Here's how the part is built. I have some questions about the finished solid (model axes, mm). Face numbers are marked on the shaded views. A direction names the side the tool comes from. Round coordinates to 2 decimals unless told otherwise and drop trailing zeros. Write each loop counter-clockwise with the first axis right and the second up, starting at its lowest first coordinate (ties: lowest second). Pieces come first, ordered by that corner, then holes. Notation, with made-up numbers: (62, 77.25) - (69, 77.25) arc R10 ccw to (69, 86.25) - close; hole circle Ø2 at (-28, 16.5). An arc over 180 degrees is marked (long way). One line per question, with ' | ' between items. Start each with the question number.
(1) Imagine slicing it at C-C (y = -6.5). Write out the boundary of the cut face in (x, z).
(2) Imagine slicing it at A-A (z = 1.7). Write out the boundary of the cut face in (x, y), plus the area to 3 significant figures.
(3) Imagine slicing it at D-D (y = -18). Write out the boundary of the cut face in (x, z), plus the area to 3 significant figures.
(4) For the marked faces 1, 2, 3 and 4, which set-ups out of +Z, -Z, +X, -X, +Y, -Y let a thin tool reach every point of the face, with its end or its side?
(5) Imagine slicing it at B-B (y = -12.5). Write out the boundary of the cut face in (x, z).
(6) If I drill on L1, parallel to Z at x = 0, y = -17.25; L2, parallel to Y at x = -1.25, z = 0.9; L3, parallel to Z at x = 3.25, y = 2, over which ranges is the centre line in solid material (lowest first)?
(7) Will these pins go through, and if not, where does the flat tip stop? pin 1 (2.5 mm diameter, centred on x = 0, y = 0, fed in from +Z); pin 2 (1 mm diameter, centred on x = -2, y = -6.5, fed in from +Z); pin 3 (1.8 mm diameter, centred on x = -1, z = -1.5, fed in from +Y); pin 4 (2 mm diameter, centred on y = -7.5, z = -1, fed in from -X).
(8) Thinking about a two-plate mould opening in Y: for the marked faces 5, 6, 7 and 8, which applies, pulls with the +Y half, pulls with the -Y half, needs draft (parallel to the pull), parting line crosses it, or undercut?
from build123d import *

# Parameters (mm, degrees)
SKETCH3_R                 = 1.4224
CUT_EXTRUDE1_DEPTH        = 3.3876
CUT_EXTRUDE1_DEPTH_BACK   = 3.3876
SKETCH4_R                 = 1.4224
BOSS_EXTRUDE1_DEPTH       = 0.79375
SKETCH5_R                 = 2.3876
BOSS_EXTRUDE2_DEPTH       = 7.9375
F_4_40_TAPPED_HOLE1_D     = 2.2606
F_4_40_TAPPED_HOLE1_DEPTH = 12.7
F_4_40_TAPPED_HOLE1_TIP   = 0.679152758


with BuildPart() as part:
    # Sketch2 → Revolve1 (revolve)
    with BuildSketch(Plane.XY):
        with BuildLine():
            Line((0, 2.3876), (0, -2.3876))
            ThreePointArc((0, -2.3876), (2.3876, 0), (0, 2.3876))
        make_face()
    revolve(axis=Axis((0, 6.043929029, 0), (0, -1, 0)))

    # Sketch3 → Cut-Extrude1 (cut, two sides)
    with BuildSketch(Plane.XY) as cut_extrude1_sk:
        Circle(SKETCH3_R)
    extrude(amount=CUT_EXTRUDE1_DEPTH, mode=Mode.SUBTRACT)
    extrude(cut_extrude1_sk.sketch, amount=-CUT_EXTRUDE1_DEPTH_BACK, mode=Mode.SUBTRACT)

    # Sketch4 → Boss-Extrude1 (add, symmetric)
    with BuildSketch(Plane.XY):
        with BuildLine():
            Line((-4.0005, 0), (-4.0005, -4.7625))
            Line((-4.0005, -4.7625), (-2.38125, -12.79525))
            Line((-2.38125, -12.79525), (2.38125, -12.79525))
            Line((2.38125, -12.79525), (4.0005, -4.7625))
            Line((4.0005, -4.7625), (4.0005, 0))
            ThreePointArc((4.0005, 0), (0, 4.0005), (-4.0005, 0))
        make_face()
        Circle(SKETCH4_R, mode=Mode.SUBTRACT)
    extrude(amount=BOSS_EXTRUDE1_DEPTH, both=True)

    # Sketch5 → Boss-Extrude2 (add, symmetric)
    with BuildSketch(Plane.XZ.offset(12.79525)):
        Circle(SKETCH5_R)
    extrude(amount=BOSS_EXTRUDE2_DEPTH, both=True)

    # #4-40 Tapped Hole1
    with Locations(Plane(origin=(0, -20.73275, 0), x_dir=(-1, 0, 0), z_dir=(0, -1, 0))):
        with Locations((0, 0)):
            Hole(F_4_40_TAPPED_HOLE1_D / 2, depth=F_4_40_TAPPED_HOLE1_DEPTH)
            with Locations((0, 0, -(F_4_40_TAPPED_HOLE1_DEPTH + F_4_40_TAPPED_HOLE1_TIP / 2))):  # 118° drill point
                Cone(0, F_4_40_TAPPED_HOLE1_D / 2, F_4_40_TAPPED_HOLE1_TIP, mode=Mode.SUBTRACT)


solid = part.part
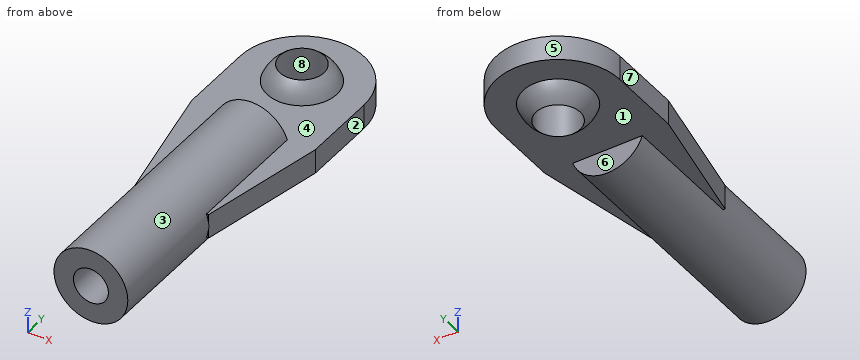
Check sheet entries:
1) outline: (-3.65, -0.79) - (-2.25, -0.79) arc R2.39 ccw to (2.25, -0.79) - (3.65, -0.79) - (3.65, 0.79) - (2.25, 0.79) arc R2.39 ccw to (-2.25, 0.79) - (-3.65, 0.79) - close
2) outline: (-1.68, -20.73) - (1.68, -20.73) - (1.68, -4.86) - (-1.68, -4.86) - close; circle Ø3.35 at (0, 0); hole circle Ø2.84 at (0, 0) | area: 55.7 mm^2
3) outline: circle Ø4.78 at (0, 0); hole circle Ø2.26 at (0, 0) | area: 13.9 mm^2
4) face 1: -Z | face 2: +Z, -Z, +X, +Y, -Y | face 3: -Y | face 4: +Z
5) outline: (-2.44, -0.79) - (-2.25, -0.79) arc R2.39 ccw to (2.25, -0.79) - (2.44, -0.79) - (2.44, 0.79) - (2.25, 0.79) arc R2.39 ccw to (-2.25, 0.79) - (-2.44, 0.79) - close; hole circle Ø2.26 at (0, 0)
6) L1: -2.39 to -1.13, 1.13 to 2.39 | L2: -20.73 to -4.86, -1.82 to -0.68, 0.68 to 1.82 | L3: -0.79 to 0.79
7) pin 1: through | pin 2: z = 1.86 | pin 3: y = 3.98 | pin 4: x = -3.65
8) face 5: pulls with the +Y half | face 6: undercut | face 7: needs draft | face 8: undercut
